Could you check a few things on this model? Use its own coordinates, in mm. Coordinates: 2 decimals unless noted, no trailing zeros. Order: outer loops, then holes, each group sorted by start corner. A loop starts at its lowest first (then second) coordinate and runs counter-clockwise, first axis right, second up. Notation, with made-up numbers: (22.5, 64) - (70.5, 64) arc R25 cw to (70.5, 89) - close; hole circle Ø10 at (-13.5, -31). An arc over 180 degrees is marked (long way). Answer as CSV lines item,"result". Start each with the question number.
1. For pin 1 (1.5 mm diameter, centred on y = -2, z = -6.5, fed in from -X); pin 2 (1.5 mm diameter, centred on x = -1, z = -5, fed in from -Y), each with a flat end and sliding along its axis, tell me the tip position at first contact or that it passes through.
2. I want a section at A-A, the plane z = 0.5. List the corners of the cut face in (x, y) for me, and give its area (3 significant figures).
3. I need wall thicknesses on probe 1 along Y at (x, z) = (0.15, -7.25); probe 2 along Y at (x, z) = (1.35, -11); probe 3 along X at (y, z) = (-1.6, -11). Which ranges of each line are inside material? Lowest first, please.
from build123d import *

# Parameters (mm, degrees)
SKETCH_1_R      = 2.5
EXTRUDE_1_DEPTH = 12.5
CHAMFER_1_SIZE  = 0.2
CHAMFER_1_SIZE2 = 0.746410162
CHAMFER_2_SIZE  = 0.2
CHAMFER_2_SIZE2 = 0.746410162


with BuildPart() as part:
    # 草图1 → 凸台-拉伸1 (new, symmetric)
    with BuildSketch(Plane.XY):
        Circle(SKETCH_1_R)
    extrude(amount=EXTRUDE_1_DEPTH, both=True)

    # 倒角1
    chamfer_1_edges = [part.edges().sort_by_distance(p)[0] for p in [
        (-2.5, 0, 12.5),
    ]]
    chamfer_1_side = [part.faces().sort_by_distance(p)[0] for p in [
        (0, 0, 12.5),
    ]]
    chamfer(chamfer_1_edges, length=CHAMFER_1_SIZE, length2=CHAMFER_1_SIZE2, reference=chamfer_1_side[0])

    # 倒角2
    chamfer_2_edges = [part.edges().sort_by_distance(p)[0] for p in [
        (-2.5, 0, -12.5),
    ]]
    chamfer_2_side = [part.faces().sort_by_distance(p)[0] for p in [
        (0, 0, -12.5),
    ]]
    chamfer(chamfer_2_edges, length=CHAMFER_2_SIZE, length2=CHAMFER_2_SIZE2, reference=chamfer_2_side[0])


solid = part.part
Solved:
1,pin 1,"stops at x = -2.17"
1,pin 2,"stops at y = -2.49"
2,outline,"circle Ø5 at (0, 0)"
2,area,"19.6 mm2"
3,probe 1,"y = -2.5 to 2.5"
3,probe 2,"y = -2.1 to 2.1"
3,probe 3,"x = -1.92 to 1.92"
